Here's the drawing with two shaded views (mm, measured from the low corner). I have some questions. Round coordinates to 2 decimals unless told otherwise and drop trailing zeros. Order: outer loops, then holes, each group sorted by start corner. A loop starts at its lowest first (then second) coordinate and runs counter-clockwise, first axis right, second up. Notation, with made-up numbers: M 72,61.25 L 131,61.25 A26 ccw 131,93.25 Z; hole C -19.75,57.25 d7. An arc over 180 degrees is marked long. One line per question, with ' | ' between items.
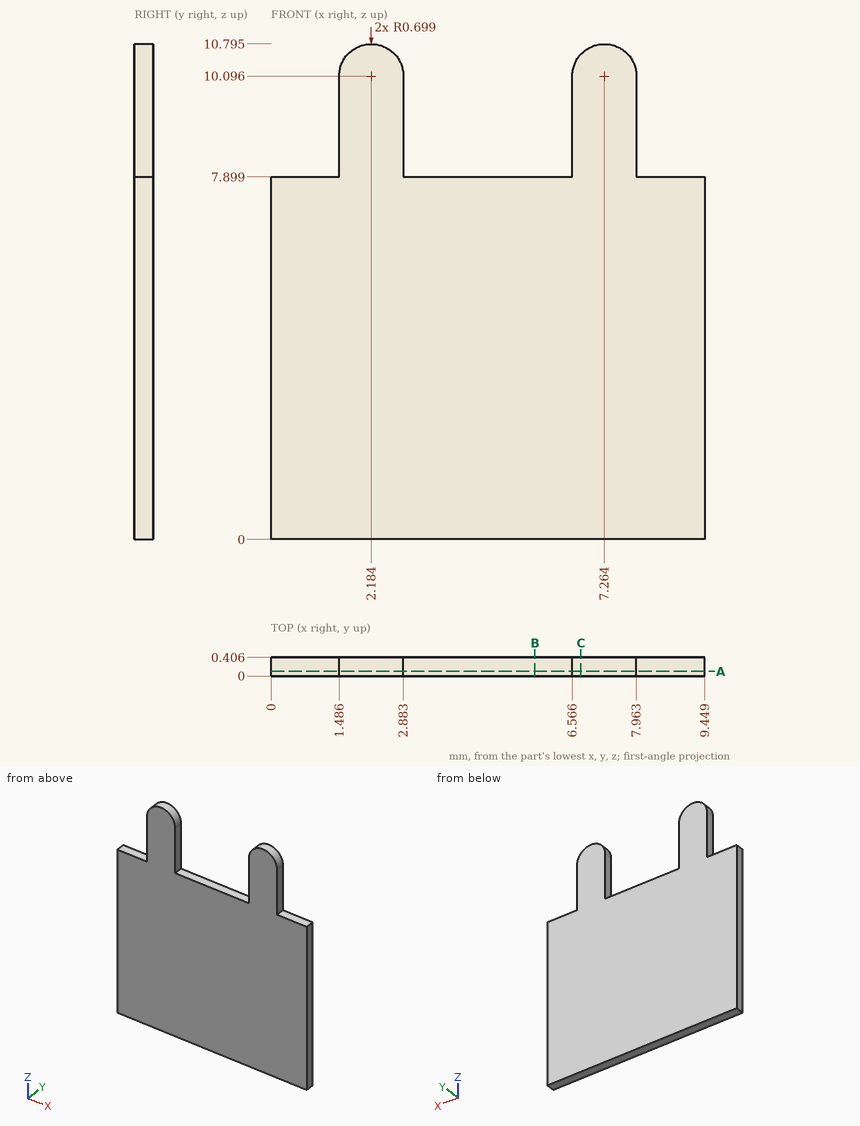
(1) If we section it at C-C on x = 6.75: Please give me the cut outline in (y, z).
Final values:
outline: M 0,0 L 0.41,0 L 0.41,10.57 L 0,10.57 Z
(2) Please list where these lines run through material, in increasing order: probe 1 along X at (y, z) = (0.1, 9.25) (1 decimal); probe 2 along Z at (x, y) = (6.5, 0.15); probe 3 along Z at (x, y) = (2.25, 0.05). Write a range as [from, to].
Final values:
probe 1: [1.5, 2.9], [6.6, 8] | probe 2: [0, 7.9] | probe 3: [0, 10.79]
(3) If we section it at A-A on y = 0.1: Please give me the cut outline in (x, z) (1 decimal).
Final values:
outline: M 0,0 L 9.4,0 L 9.4,7.9 L 8,7.9 L 8,10.1 A0.7 ccw 6.6,10.1 L 6.6,7.9 L 2.9,7.9 L 2.9,10.1 A0.7 ccw 1.5,10.1 L 1.5,7.9 L 0,7.9 Z
(4) Will this pin go through, and if not, where does the flat tip stop? pin 1 Ø5 at (x, z) = (7.5, 2.5) entering from -Y.
Final values:
pin 1: y = 0
(5) If we section it at B-B on x = 5.75: Please give me the cut outline in (y, z).
Final values:
outline: M 0,0 L 0.41,0 L 0.41,7.9 L 0,7.9 Z
